Geometry check sheet. Reference: drawing and pictorial views, mm from the part's lowest x, y, z. Give positions to 0.01 mm unless a question says otherwise; leave off trailing zeros. Order: outer loops, then holes, each group sorted by start corner. A loop starts at its lowest first (then second) coordinate and runs counter-clockwise, first axis right, second up. Notation, with made-up numbers: (-39, 40.5) - (9, 40.5) arc R10 cw to (9, 54.5) - close; hole circle Ø7 at (4.5, 62.5). An arc over 180 degrees is marked (long way). Answer as a JSON object with one key per item and string values.
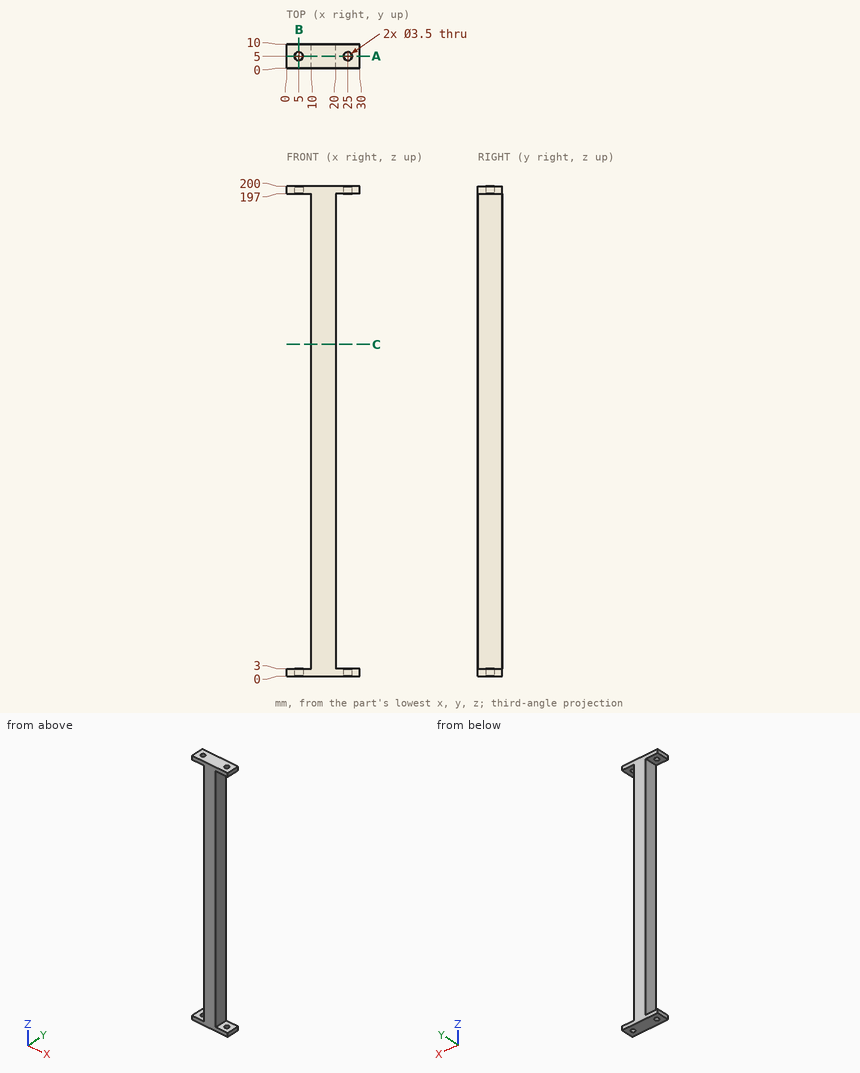
(1) Gauge pin test, flat ends, axial feed: pin 1 Ø5 at (y, z) = (5, 101.5) entering from +X; pin 2 Ø1 at (y, z) = (2.5, 49) entering from -X. Record the tip position at first contact, or that the pin passes through.
Computed values:
{"pin 1": "stops at x = 20", "pin 2": "stops at x = 10"}
(2) Section check B-B (x = 5). Record the cut outline in (y, z), then the cut area to 3 significant figures.
Computed values:
{"outline": "(0, 0) - (3.25, 0) - (3.25, 3) - (0, 3) - close; (0, 197) - (3.25, 197) - (3.25, 200) - (0, 200) - close; (6.75, 0) - (10, 0) - (10, 3) - (6.75, 3) - close; (6.75, 197) - (10, 197) - (10, 200) - (6.75, 200) - close", "area": "39.0 mm²"}
(3) Section check C-C (z = 135.5). Record the cut outline in (x, y), then the cut area to 3 significant figures.
Computed values:
{"outline": "(10, 0) - (20, 0) - (20, 10) - (10, 10) - close", "area": "100 mm²"}
(4) Material ranges on line 1 along X through (y, z) = (5, 1); line 2 along Z through (x, y) = (2.5, 3.5); line 3 along Y through (x, z) = (25, 198.35), recorded low to high. Write a range as [from, to].
Computed values:
{"line 1": "x = [0, 3.25], [6.75, 23.25], [26.75, 30]", "line 2": "z = [0, 3], [197, 200]", "line 3": "y = [0, 3.25], [6.75, 10]"}
(5) Section check A-A (y = 5). Record the cut outline in (x, z).
Computed values:
{"outline": "(0, 0) - (3.25, 0) - (3.25, 3) - (0, 3) - close; (0, 197) - (3.25, 197) - (3.25, 200) - (0, 200) - close; (6.75, 0) - (23.25, 0) - (23.25, 3) - (20, 3) - (20, 197) - (23.25, 197) - (23.25, 200) - (6.75, 200) - (6.75, 197) - (10, 197) - (10, 3) - (6.75, 3) - close; (26.75, 0) - (30, 0) - (30, 3) - (26.75, 3) - close; (26.75, 197) - (30, 197) - (30, 200) - (26.75, 200) - close"}
